Geometry: final body of the model. Coordinates: model frame, mm. A direction names the side the tool comes from. Give positions to 0.01 mm unless a question says otherwise; leave off trailing zeros. Loops run counter-clockwise (first coordinate to the right, second up) from the corner with the lowest first, then second, coordinate; pieces in that order, holes last.
Autodesk Inventor part; units mm, degrees
ref_plane "YZ Plane" through (0, 0, 0) normal (1, 0, 0) x (0, 1, 0)
ref_plane "XZ Plane" through (0, 0, 0) normal (0, 1, 0) x (-1, 0, 0)
ref_plane "XY Plane" through (0, 0, 0) normal (0, 0, 1) x (1, 0, 0)
sketch "スケッチ1" plane through (0, 0, 0) normal (0, 0, 1) x (1, 0, 0)
  circle A0 centre (0, 0) radius 10
  line L0 (0, 0) -> (7.5, 0)
  line L1 (7.5, 0) -> (7.5, -45)
  line L2 (7.5, -45) -> (-2.5, -45)
  line L3 (-2.5, -45) -> (-2.5, 0)
  circle A1 centre (2.5, -22) radius 1.7
  circle A2 centre (2.5, -32) radius 1.7
  circle A3 centre (2.5, -42) radius 1.7
  circle A4 centre (0, 0) radius 5.5
  circle A5 centre (0, 5.5) radius 1.25
  circle A6 centre (0, -5.5) radius 1.25
  circle A7 centre (0, 0) radius 2
  line L4 (0, 0) -> (0, -45)
  point P0 (7.5, -6.6144)
  point P1 (-2.5, -9.6825)
  dimension "d0" = 20
  dimension "d3" = 7.5
  dimension "d4" = 45
  dimension "d5" = 10
  dimension "d6" = 3.4
  dimension "d7" = 3.4
  dimension "d8" = 3.4
  dimension "d9" = 11
  dimension "d10" = 2.5
  dimension "d11" = 2.5
  dimension "d12" = 4
  dimension "d16" = 2.5
  dimension "d17" = 2.5
  dimension "d18" = 2.5
extrude "押し出し1" add sketch "スケッチ1" along normal blind 2 contours A0 L1 L0 A4 A5 L3 | L3 A4 A6 L4 A0 | A0 L4 L2 L3 | L1 L2 L4 A0 | A0 L4 A6 A4 L0 L1 | A4 A5 L0 A7 L4 A6 | A4 A6 L4 A7 L0
fillet "フィレット1" radius 2 2 edges at (7.5, -6.6144, 1) (-2.5, -9.6825, 1)
properties part number "cutter_board_claws_endeffector_8_5_rotary-blade"
Item 1: Set-up query: faces 5 (the face through (3, -45, 1)), 6 (the face through (7.5, -26, 1)), 7 (the face through (-2.5, -28, 1)). Return all of +Z, -Z, +X, -X, +Y, -Y with unobstructed straight access to the full face (end or side cutting, diameter ignored); none if empty.
Values follow:
face 5: +Z, -Z, +X, -X, -Y
face 6: +Z, -Z, +X, -Y
face 7: +Z, -Z, -X, -Y
Item 2: Section query D-D on y = 0. Return loops of the section in (x, z), plus the area to 3 significant figures.
Values follow:
outline: (-10, 0) - (-2, 0) - (-2, 2) - (-10, 2) - close; (2, 0) - (10, 0) - (10, 2) - (2, 2) - close
area: 32.0 mm2
Item 3: Section query A-A on y = -42. Return loops of the section in (x, z), plus the area to 3 significant figures.
Values follow:
outline: (-2.5, 0) - (0.8, 0) - (0.8, 2) - (-2.5, 2) - close; (4.2, 0) - (7.5, 0) - (7.5, 2) - (4.2, 2) - close
area: 13.2 mm2
Item 4: Pin query (flat end, axial travel): pin 1 (1 mm diameter, centred on y = -16.5, z = 1, fed in from -X); pin 2 (1 mm diameter, centred on x = 7.5, z = 1, fed in from +Y); pin 3 (2 mm diameter, centred on x = 2.5, y = -42, fed in from +Z); pin 4 (1 mm diameter, centred on y = -19.5, z = 1, fed in from +X). Return the tip coordinate at first contact, or that it passes through.
Values follow:
pin 1: stops at x = -2.5
pin 2: stops at y = 7.14
pin 3: passes through
pin 4: stops at x = 7.5
Item 5: Section query B-B on z = 0.4. Return loops of the section in (x, y).
Values follow:
outline: (-3.75, -9.27) arc R2 cw to (-2.5, -11.12) - (-2.5, -45) - (7.5, -45) - (7.5, -7.33) arc R2 cw to (7.92, -6.11) arc R10 ccw (long way) to start; hole circle Ø4 at (0, 0); hole circle Ø2.5 at (0, -5.5); hole circle Ø2.5 at (0, 5.5); hole circle Ø3.4 at (2.5, -42); hole circle Ø3.4 at (2.5, -32); hole circle Ø3.4 at (2.5, -22)
Item 6: Draft query along X for faces 1 (the face through (-2.95, 9.555, 0.986)), 2 (the face through (2, -17, 0)), 3 (the face through (3.414, -23.433, 0.986)), 4 (the face through (3.3, -40.5, 1)). Return one class per face: +X half, -X half, draft (parallel to the pull), parting line (faces both ways), or undercut.
Values follow:
face 1: parting line
face 2: draft
face 3: undercut
face 4: undercut
Item 7: Section query C-C on x = 3.25. Return loops of the section in (y, z).
Values follow:
outline: (-45, 0) - (-43.53, 0) - (-43.53, 2) - (-45, 2) - close; (-40.47, 0) - (-33.53, 0) - (-33.53, 2) - (-40.47, 2) - close; (-30.47, 0) - (-23.53, 0) - (-23.53, 2) - (-30.47, 2) - close; (-20.47, 0) - (9.46, 0) - (9.46, 2) - (-20.47, 2) - close
Item 8: Ray query, probe 1 along Y at (x, z) = (0, 0.55); probe 2 along Y at (x, z) = (-1, 1.7); probe 3 along X at (y, z) = (-43, 0.2). Return the intervals inside material, ascending.
Values follow:
probe 1: y = -45 to -6.75, -4.25 to -2, 2 to 4.25, 6.75 to 10
probe 2: y = -45 to -6.25, -4.75 to -1.73, 1.73 to 4.75, 6.25 to 9.95
probe 3: x = -2.5 to 1.13, 3.87 to 7.5
